Model file for the job. Use its own axes, mm. Face numbers are marked on the shaded views. A direction names the side the tool comes from. Give positions to 0.01 mm unless a question says otherwise; leave off trailing zeros. Loops run counter-clockwise (first coordinate to the right, second up) from the corner with the lowest first, then second, coordinate; pieces in that order, holes last. Notation, with made-up numbers: (29, 27) - (50, 27) arc R12 cw to (50, 34) - close; hole circle Ø1 at (15, 53). An arc over 180 degrees is marked (long way). Answer as CSV lines item,"result". Start each with the question number.
Item 1: Saw through at A-A on z = 11.75. Give the cut face in (x, y), plus the area to 4 significant figures.
Item 2: Saw through at C-C on x = 17.75. Give the cut face in (y, z), plus the area to 4 significant figures.
Item 3: Tool access for the marked faces 1, 2, 3 and 4: list every direction of +Z, -Z, +X, -X, +Y, -Y with a clear straight run to the whole face (end or side of a thin tool).
Item 4: Drill centre lines: L1, parallel to Y at x = 8.5, z = 4.75; L2, parallel to X at y = -4.25, z = 14.5; L3, parallel to Y at x = 1.75, z = 14. Where is each one in solid material? Low to high. Write a range as from..to.
Item 5: Saw through at B-B on x = 10.75. Give the cut face in (y, z), plus the area to 4 significant figures.
Item 6: Pull direction Y, two halves, no side cores. Call the marked faces 5, 6, 7 and 8: pulls with the +Y half, pulls with the -Y half, needs draft (parallel to the pull), parting line crosses it, or undercut.
Item 7: Pin check, flat tips, straight feed: pin 1 (1.6 mm diameter, centred on x = -1, z = 5, fed in from +Y); pin 2 (10 mm diameter, centred on x = 13.5, z = 8.5, fed in from +Y); pin 3 (4 mm diameter, centred on x = 10, y = -9, fed in from -Z); pin 4 (0.8 mm diameter, centred on y = -8, z = -1, fed in from +X). Stop position of each tip, or through.
from build123d import *

# Parameters (mm, degrees)
F0_W     = 2.5
F0_H     = 8
F0_W_2   = 8
F0_H_2   = 2.5
F1_DEPTH = 17
F2_START = 2.5
F2_DEPTH = 12
F3_START = 5.5
F3_DEPTH = 6
F4_R     = 2.99999
F5_START = 6.5
F0_W_3   = 1.5
F0_H_3   = 1.5
F5_DEPTH = 4


# Not quite as in the source:
# - a fillet or chamfer is up to 0.001 mm smaller than in the source, because OpenCascade refuses the exact size


with BuildPart() as f1:
    # F0 (on Front) → F1 (new body)
    with BuildSketch(Plane.XZ):
        Polygon((20, 2.5), (2.5, 20), (2.5, 15.25), (2.5, 7.25), (2.5, 2.5), (7.25, 2.5), (15.25, 2.5), align=None)
        Polygon((20, 0), (20, 2.5), (15.25, 2.5), (15.25, 0), (16.5, 0), (19, 0), align=None)
        Polygon((2.5, 20), (0, 20), (0, 19), (0, 16.5), (0, 15.25), (2.5, 15.25), align=None)
        Polygon((2.5, 2.5), (2.5, 7.25), (0, 7.25), (0, 6), (0, 3.5), (0, 0), (3.5, 0), (6, 0), (7.25, 0), (7.25, 2.5), align=None)
        with Locations((1.25, 11.25)):
            Rectangle(F0_W, F0_H)
        with Locations((11.25, 1.25)):
            Rectangle(F0_W_2, F0_H_2)
    extrude(amount=F1_DEPTH)

    # F0 (on Front) → F2 (cut)
    with BuildSketch(Plane.XZ.offset(F2_START)):
        Polygon((20, 2.5), (2.5, 20), (2.5, 15.25), (2.5, 7.25), (2.5, 2.5), (7.25, 2.5), (15.25, 2.5), align=None)
    extrude(amount=F2_DEPTH, mode=Mode.SUBTRACT)

    # F0 (on Front) → F3 (cut)
    with BuildSketch(Plane.XZ.offset(F3_START)):
        with Locations((1.25, 11.25)):
            Rectangle(F0_W, F0_H)
        with Locations((11.25, 1.25)):
            Rectangle(F0_W_2, F0_H_2)
    extrude(amount=F3_DEPTH, mode=Mode.SUBTRACT)

    # F4 (radius 3 in the source; OpenCascade refuses exactly that, so slightly less here)
    f4_edges = [f1.edges().sort_by_distance(p)[0] for p in [
        (1.25, -11.5, 7.25),
        (1.25, -5.5, 7.25),
        (1.25, -11.5, 15.25),
        (1.25, -5.5, 15.25),
        (7.25, -11.5, 1.25),
        (7.25, -5.5, 1.25),
        (15.25, -11.5, 1.25),
        (15.25, -5.5, 1.25),
    ]]
    fillet(f4_edges, radius=F4_R)

    # F0 (on Front) → F5 (join)
    with BuildSketch(Plane.XZ.offset(F5_START)):
        with Locations((-0.75, 17.75)):
            Rectangle(F0_W_3, F0_H_2)
        with Locations((-0.75, 4.75)):
            Rectangle(F0_W_3, F0_H_2)
        with Locations((4.75, -0.75)):
            Rectangle(F0_W, F0_H_3)
        with Locations((17.75, -0.75)):
            Rectangle(F0_W, F0_H_3)
    extrude(amount=F5_DEPTH)


solid = f1.part
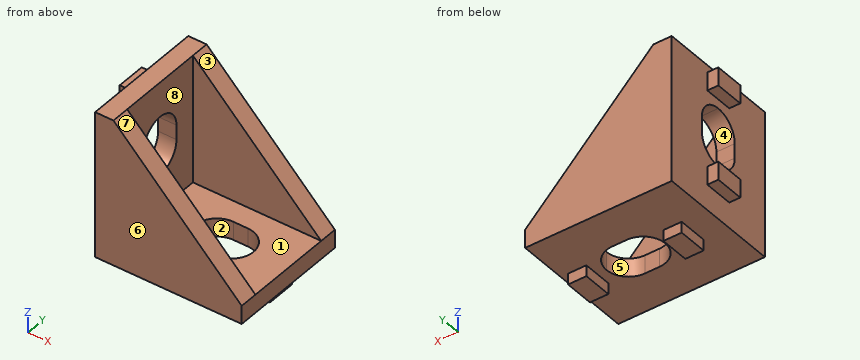
Responses:
1,outline,"(0, -17) - (10.75, -17) - (10.75, -14.5) - (2.5, -14.5) - (2.5, -11.5) - (0, -11.5) - close; (0, -5.5) - (2.5, -5.5) - (2.5, -2.5) - (10.75, -2.5) - (10.75, 0) - (0, 0) - close"
1,area,"68.75 mm2"
2,outline,"(-17, 0) - (-10.5, 0) - (-10.5, -1.5) - (-6.5, -1.5) - (-6.5, 0) - (0, 0) - (0, 4.75) - (-2.5, 4.75) - (-2.5, 2.5) - (-14.5, 2.5) - (-14.5, 4.75) - (-17, 4.75) - close"
2,area,"59.75 mm2"
3,face 1,"+Z, +X"
3,face 2,"+Z, -Z"
3,face 3,"+Z, +X, +Y, -Y"
3,face 4,"+X, -X"
4,L1,"-17..-14.5, -2.5..0"
4,L2,"0..2.5"
4,L3,"-17..-10.94, -6.06..0"
5,outline,"(-17, 0) - (-11.5, 0) - (-11.5, 2.5) - (-14.5, 2.5) - (-14.5, 11.75) - (-17, 11.75) - close; (-5.5, 0) - (0, 0) - (0, 11.75) - (-2.5, 11.75) - (-2.5, 2.5) - (-5.5, 2.5) - close"
5,area,"73.75 mm2"
6,face 5,"undercut"
6,face 6,"pulls with the -Y half"
6,face 7,"needs draft"
6,face 8,"undercut"
7,pin 1,"y = -6.5"
7,pin 2,"y = 0"
7,pin 3,"through"
7,pin 4,"x = 19"
